Source: CAD feature listing. Evaluate the final solid. Frame: model axes, mm. A direction names the side the tool comes from. Coordinates: 2 decimals unless noted, no trailing zeros. Write each loop counter-clockwise with the first axis right and the second up, starting at its lowest first coordinate (ties: lowest second). Pieces come first, ordered by that corner, then holes. Notation, with made-up numbers: (-9.5, 47) -> (35.5, 47) arc R16 ccw to (35.5, 68) -> close; hole circle Ø4 at (3.5, 61). An arc over 180 degrees is marked (long way). One line per item, written item: value. Start each with the question number.
1. Line query: line 1 (Y direction, x = -6, z = 194); line 2 (Z direction, x = 0, y = -2.5); line 3 (Z direction, x = -4, y = -29.5). Output: solid intervals per line, ascending.
2. Access query for faces 1 (the cylindrical face through (-7.493, 25.446, 955.33)), 2 (the cylindrical face through (-7.493, -25.848, 955.33)), 3 (the conical face through (21.493, -6.553, 266.178)), 4 (the flat face through (0, 40, 955)). Directions: +Z, -Z, +X, -X, +Y, -Y. A direction counts if a zero-diameter tool reaches every point of the face in a straight line with its end or side. Return the directions, or none.
3. Mould query, pull axis Z, two halves, no side actions, for faces 5 (the cylindrical face through (-7.493, -30.438, 20.33)), 6 (the flat face through (0, 40, 20)), 7 (the conical face through (3, 1, 975)). Classes: released by +Z, released by -Z, zero draft, split by the parting line, or undercut.
4. Section query A-A, the plane y = -31. Output: boundary loops of the cut face in (x, z), and give its area (3 significant figures).
5. First-contact query: P1, Ø4, axis at x = -10, y = 0.5, coming from the -Z side; P2, Ø1.5, axis at x = 6.5, z = 317.5, coming from the -Y side; P3, Ø10, axis at x = -15.5, z = 467, coming from the -Y side. Flat tips, straight axial feed; report the tip coordinate or a pass-through.
from build123d import *

# Parameters (mm, degrees)
F2_R     = 7.5
F3_DEPTH = 40


with BuildPart() as f1:
    # F0 (on Front) → F1 (revolve)
    with BuildSketch(Plane.XZ):
        Polygon((2.5, 975), (0, 0), (22.5, 0), (22.5, 525), (17.5, 525), (17.5, 975), align=None)
    revolve(axis=Axis((1.25, 0, 487.5), (-0.0025640941, 0, -0.9999967127)))

    # F2 (on Front) → F3 (join, symmetric)
    with BuildSketch(Plane.XZ):
        with Locations((0, 20)):
            Circle(F2_R)
        with Locations((0, 955)):
            Circle(F2_R)
    extrude(amount=F3_DEPTH, both=True)


solid = f1.part
Computed values:
1. line 1: y = -21.02 to 21.02
1. line 2: z = 0.01 to 975.02
1. line 3: z = 13.66 to 26.34, 948.66 to 961.34
2. face 1: +Y
2. face 2: -Y
2. face 3: none
2. face 4: +Z, -Z, +X, -X, +Y
3. face 5: undercut
3. face 6: zero draft
3. face 7: released by +Z
4. outline: circle Ø15 at (0, 20); circle Ø15 at (0, 955)
4. area: 353 mm²
5. P1: stops at z = 0.04
5. P2: stops at y = -21.12
5. P3: stops at y = -17.8
